```python
from build123d import *

# Parameters (mm, degrees)
SKETCH1_W           = 3
SKETCH1_H           = 15
BOSS_EXTRUDE1_DEPTH = 3
SKETCH3_W           = 36
SKETCH3_H           = 15
BOSS_EXTRUDE2_DEPTH = 3
SKETCH4_R           = 5
SKETCH4_R_2         = 1.5
CUT_EXTRUDE1_DEPTH  = 37.742346142
SKETCH5_R           = 0.8
CUT_EXTRUDE2_DEPTH  = 37.742346142
FILLET1_R           = 2


with BuildPart() as part:
    # Sketch1 → Boss-Extrude1 (new body)
    with BuildSketch(Plane.XY):
        Polygon((-18, -7.5), (-18, -15), (18, -15), (18, -7.5), (15, -7.5), (15, 7.5), (18, 7.5), (18, 15), (-18, 15), (-18, 7.5), (-15, 7.5), (-15, -7.5), align=None)
        with Locations((-19.5, 0)):
            Rectangle(SKETCH1_W, SKETCH1_H)
        with Locations((-16.5, 0)):
            Rectangle(SKETCH1_W, SKETCH1_H)
        with Locations((19.5, 0)):
            Rectangle(SKETCH1_W, SKETCH1_H)
        with Locations((16.5, 0)):
            Rectangle(SKETCH1_W, SKETCH1_H)
    extrude(amount=BOSS_EXTRUDE1_DEPTH)

    # Sketch3 → Boss-Extrude2 (add)
    with BuildSketch(Plane(origin=(0, 0, 0), x_dir=(-1, 0, 0), z_dir=(0, 0, -1))):
        with Locations((0, 22.5)):
            Rectangle(SKETCH3_W, SKETCH3_H)
    extrude(amount=-BOSS_EXTRUDE2_DEPTH)

    # Sketch4 → Cut-Extrude1 (cut, through all)
    with BuildSketch(Plane(origin=(0, 0, 0), x_dir=(-1, 0, 0), z_dir=(0, 0, -1))):
        with Locations((0, 7)):
            Circle(SKETCH4_R)
        with Locations((-8.5, 7)):
            Circle(SKETCH4_R_2)
        with Locations(Location((8.5, 7, 0), (0, 0, 180))):
            Circle(SKETCH4_R_2)
    extrude(amount=-CUT_EXTRUDE1_DEPTH, mode=Mode.SUBTRACT)

    # Sketch5 → Cut-Extrude2 (cut, through all)
    with BuildSketch(Plane(origin=(0, 0, 0), x_dir=(-1, 0, 0), z_dir=(0, 0, -1))):
        with Locations((-18, 7.5)):
            Circle(SKETCH5_R)
        with Locations((-18, -7.5)):
            Circle(SKETCH5_R)
        with Locations((18, 7.5)):
            Circle(SKETCH5_R)
        with Locations((18, -7.5)):
            Circle(SKETCH5_R)
    extrude(amount=-CUT_EXTRUDE2_DEPTH, mode=Mode.SUBTRACT)

    # Fillet1
    fillet1_edges = [part.edges().sort_by_distance(p)[0] for p in [
        (18, -15, 1.5),
        (-18, -15, 1.5),
        (-18, 30, 1.5),
        (18, 30, 1.5),
    ]]
    fillet(fillet1_edges, radius=FILLET1_R)


solid = part.part
```
Check sheet for the modelled part. Datum: model origin and axes. Units: mm. A direction names the side the tool comes from. Give positions to 0.01 mm unless a question says otherwise; leave off trailing zeros. Order: outer loops, then holes, each group sorted by start corner. A loop starts at its lowest first (then second) coordinate and runs counter-clockwise, first axis right, second up. Notation, with made-up numbers: (68, 70.5) -> (116, 70.5) arc R23 cw to (116, 92.5) -> close; hole circle Ø8 at (10.5, 33). An arc over 180 degrees is marked (long way). Use CSV: the item, a comma, the result in double quotes. Start each with the question number.
1) Mould release check, pull along Y, two halves, no side actions. Record for faces 1 (the face through (-20, 7.5, 1)), 2 (the face through (-17.45, -6.92, 1.48)), 3 (the face through (17.45, 6.92, 1.48)), 4 (the face through (-20, -7.5, 1)): released by +Y, released by -Y, zero draft, split by the parting line, or undercut.
2) Sectioned sample at B-B, the plane z = 1.75. Record the boundary of the cut face in (x, y), plus the area to 3 significant figures.
3) Sectioned sample at A-A, the plane x = 8.5. Record the boundary of the cut face in (y, z), plus the area to 3 significant figures.
4) Sectioned sample at D-D, the plane y = 16. Record the boundary of the cut face in (x, z), plus the area to 3 significant figures.
5) Go/stop test with flat-tipped pins: P1, Ø1.1, axis at x = -20.5, z = 1, coming from the -Y side; P2, Ø1.3, axis at x = -18, y = 7.5, coming from the +Z side; P3, Ø0.7, axis at x = 20.5, z = 2, coming from the +Y side; P4, Ø2, axis at x = 13, y = -7, coming from the -Z side. Record where each tip stops, or that it passes through.
6) Set-up check for faces 5 (the face through (20, -7.5, 1)), 6 (the face through (-18, -11, 1)), 7 (the face through (21, 0, 1)), 8 (the face through (20, 7.5, 1)), 9 (the face through (9.7, 6.1, 1.5)): record each of +Z, -Z, +X, -X, +Y, -Y from which the full face is reachable in a straight line by a thin tool's end or side.
7) Sectioned sample at C-C, the plane x = 0. Record the boundary of the cut face in (y, z), plus the area to 3 significant figures.
8) Material ranges on line 1 (X direction, y = 8, z = 0.55); line 2 (Y direction, x = 8.5, z = 0.8); line 3 (X direction, y = 19, z = 1.3), recorded low to high. Write a range as from..to.
Recorded:
1,face 1,"released by +Y"
1,face 2,"undercut"
1,face 3,"undercut"
1,face 4,"released by -Y"
2,outline,"(-21, -7.5) -> (-18.8, -7.5) arc R0.8 cw (long way) to (-18, -8.3) -> (-18, -13) arc R2 ccw to (-16, -15) -> (16, -15) arc R2 ccw to (18, -13) -> (18, -8.3) arc R0.8 cw (long way) to (18.8, -7.5) -> (21, -7.5) -> (21, 7.5) -> (18.8, 7.5) arc R0.8 cw (long way) to (18, 8.3) -> (18, 28) arc R2 ccw to (16, 30) -> (-16, 30) arc R2 ccw to (-18, 28) -> (-18, 8.3) arc R0.8 cw (long way) to (-18.8, 7.5) -> (-21, 7.5) -> close; hole circle Ø3 at (-8.5, 7); hole circle Ø10 at (0, 7); hole circle Ø3 at (8.5, 7)"
2,area,"1,610 mm2"
3,outline,"(-15, 0) -> (5.5, 0) -> (5.5, 3) -> (-15, 3) -> close; (8.5, 0) -> (30, 0) -> (30, 3) -> (8.5, 3) -> close"
3,area,"126 mm2"
4,outline,"(-18, 0) -> (18, 0) -> (18, 3) -> (-18, 3) -> close"
4,area,"108 mm2"
5,P1,"y = -7.5"
5,P2,"through"
5,P3,"y = 7.5"
5,P4,"z = 0"
6,face 5,"+Z, -Z, +X, -Y"
6,face 6,"+Z, -Z, -X, -Y"
6,face 7,"+Z, -Z, +X, +Y, -Y"
6,face 8,"+Z, -Z, +X, +Y"
6,face 9,"+Z, -Z"
7,outline,"(-15, 0) -> (2, 0) -> (2, 3) -> (-15, 3) -> close; (12, 0) -> (30, 0) -> (30, 3) -> (12, 3) -> close"
7,area,"105 mm2"
8,line 1,"-17.38..-9.62, -7.38..-4.9, 4.9..7.38, 9.62..17.38"
8,line 2,"-15..5.5, 8.5..30"
8,line 3,"-18..18"
